Design review of the part built by this model. Coordinates are the model's own, in mm. Give positions to 0.01 mm unless a question says otherwise; leave off trailing zeros. Write each loop counter-clockwise with the first axis right and the second up, starting at its lowest first coordinate (ties: lowest second). Pieces come first, ordered by that corner, then holes. Notation, with made-up numbers: (42, 24.5) -> (48, 24.5) arc R20 ccw to (48, 49.5) -> close; hole circle Ø1 at (20, -14.5). An arc over 180 degrees is marked (long way). Write each question's results on one line, items separated by ' | '. Start each with the question number.
(1) Take a section at C-C (z = 15). State the section outline as (x, y) points, plus the area to 3 significant figures.
(2) Take a section at A-A (x = 0). State the section outline as (y, z) points, plus the area to 3 significant figures.
(3) Clearance check with flat-ended pins moving along their axes: pin 1 (1 mm diameter, centred on y = 2, z = 6.5, fed in from +X); pin 2 (1.5 mm diameter, centred on x = 2, z = 3.5, fed in from +Y). State where each tip first meets the part, or that it passes through.
(4) To check wall thickness, follow probe 1 along Y at (x, z) = (0, -5.5); probe 2 along Y at (x, z) = (0.4, -9). State the ranges of each line that lie inside material, in increasing order.
from build123d import *

# Parameters (mm, degrees)
F0_R     = 2.8829
F1_DEPTH = 17.5
F2_R     = 1.49987
F3_DEPTH = 35.001
F4_SIZE  = 0.254


with BuildPart() as f1:
    # F0 (on Top) → F1 (new body, symmetric)
    with BuildSketch(Plane.XY):
        Circle(F0_R)
    extrude(amount=F1_DEPTH, both=True)

    # F2 (on face) → F3 (cut, through all)
    with BuildSketch(Plane.XY.offset(17.5)):
        Circle(F2_R)
    extrude(amount=-F3_DEPTH, mode=Mode.SUBTRACT)

    # F4
    f4_edges = [f1.edges().sort_by_distance(p)[0] for p in [
        (-1.49987, 0, 17.5),
        (-1.49987, 0, -17.5),
    ]]
    chamfer(f4_edges, length=F4_SIZE)


solid = f1.part
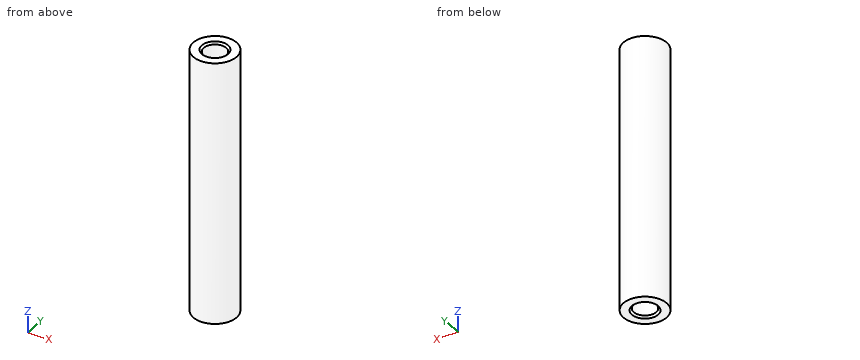
Report:
1) outline: circle Ø5.77 at (0, 0); hole circle Ø3 at (0, 0) | area: 19.0 mm2
2) outline: (-2.88, -17.5) -> (-1.75, -17.5) -> (-1.5, -17.25) -> (-1.5, 17.25) -> (-1.75, 17.5) -> (-2.88, 17.5) -> close; (1.5, -17.25) -> (1.75, -17.5) -> (2.88, -17.5) -> (2.88, 17.5) -> (1.75, 17.5) -> (1.5, 17.25) -> close | area: 96.7 mm2
3) pin 1: x = 2.46 | pin 2: y = 2.6
4) probe 1: -2.88 to -1.5, 1.5 to 2.88 | probe 2: -2.86 to -1.45, 1.45 to 2.86
